```python
from build123d import *

# Parameters (mm, degrees)
SKETCH1_R           = 5
BOSS_EXTRUDE1_DEPTH = 10
SKETCH3_R           = 15
CUT_EXTRUDE2_DEPTH  = 2.5
SKETCH4_R           = 5
CUT_EXTRUDE3_DEPTH  = 74.484692283


with BuildPart() as part:
    # Sketch1 → Boss-Extrude1 (new, symmetric)
    with BuildSketch(Plane.XY):
        with BuildLine():
            Line((0, 10), (60, 10))
            ThreePointArc((60, 10), (70, 0), (60, -10))
            Line((60, -10), (0, -10))
            ThreePointArc((0, -10), (-10, 0), (0, 10))
        make_face()
        Circle(SKETCH1_R, mode=Mode.SUBTRACT)
        with Locations((60, 0)):
            Circle(SKETCH1_R, mode=Mode.SUBTRACT)
    extrude(amount=BOSS_EXTRUDE1_DEPTH, both=True)

    # Sketch3 → Cut-Extrude2 (cut, symmetric)
    with BuildSketch(Plane.XY):
        Circle(SKETCH3_R)
        with Locations((60, 0)):
            Circle(SKETCH3_R)
    extrude(amount=CUT_EXTRUDE2_DEPTH, both=True, mode=Mode.SUBTRACT)

    # Sketch4 → Cut-Extrude3 (cut, through all)
    with BuildSketch(Plane(origin=(0, 10, 0), x_dir=(1, 0, 0), z_dir=(0, 1, 0))):
        with Locations(Location((30, 0, 0), (0, 0, 270))):
            Circle(SKETCH4_R)
    extrude(amount=-CUT_EXTRUDE3_DEPTH, mode=Mode.SUBTRACT)


solid = part.part
```
Geometry check sheet. Reference: the model listing, model coordinates, mm. A direction names the side the tool comes from. Round coordinates to 2 decimals unless told otherwise and drop trailing zeros. Loops run counter-clockwise (first coordinate to the right, second up) from the corner with the lowest first, then second, coordinate; pieces in that order, holes last. Notation, with made-up numbers: (78, 41) - (84, 41) arc R27 cw to (84, 65) - close; hole circle Ø9 at (65.5, 72.5). An arc over 180 degrees is marked (long way). Write item = value, one per line. Start each with the question number.
1. Section check C-C on z = 0. Enter the section's corners in (x, y).
2. Section check B-B on x = 53.5. Enter the section's corners in (y, z).
3. Section check A-A on y = 0. Give the number of separate pieces and of enclosed holes in the cut face, then the cut area to 3 significant figures.
4. Section check D-D on z = -7.5. Enter the section's corners in (x, y), then the cut area to 3 significant figures.
5. Depth check by flat-ended pin: pin 1 (8 mm diameter, centred on y = 6, z = -4, fed in from +X); pin 2 (6 mm diameter, centred on x = 0, y = 0, fed in from +Z); pin 3 (8 mm diameter, centred on y = -4.5, z = -1.5, fed in from +X); pin 4 (8 mm diameter, centred on y = -7.5, z = -2, fed in from +X). Enter the tip coordinate at first touch or a pass-through.
6. Mould release check, pull along X, two halves, no side actions. Record for faces 3 (the face through (55, 0, 6)), 4 (the face through (15, 0, 0)), 5 (the face through (54.5, 0.1, -2.5)): released by +X, released by -X, zero draft, split by the parting line, or undercut.
7. Set-up check for faces 1 (the face through (-1.08, -4.88, -6.3)), 2 (the face through (45, 0, 0)): record each of +Z, -Z, +X, -X, +Y, -Y from which the full face is reachable in a straight line by a thin tool's end or side.
8. Thickness scan on line 1 (Z direction, x = 6.5, y = -4.75); line 2 (X direction, y = 0, z = -7); line 3 (Y direction, x = 0, z = -4.75). Record the ranges inside material, lowest first.
Working result:
q1.outline = (11.18, -10) - (25, -10) - (25, 10) - (11.18, 10) arc R15 cw to start; (35, -10) - (48.82, -10) arc R15 cw to (48.82, 10) - (35, 10) - close
q2.outline = (-10, -10) - (10, -10) - (10, -2.5) - (-10, -2.5) - close; (-10, 2.5) - (10, 2.5) - (10, 10) - (-10, 10) - close
q3.separate_pieces = 5
q3.enclosed_holes = 1
q3.area = 971 mm^2
q4.outline = (0, -10) - (60, -10) arc R10 ccw to (60, 10) - (0, 10) arc R10 ccw to start; hole circle Ø10 at (0, 0); hole circle Ø10 at (60, 0)
q4.area = 1,360 mm^2
q5.pin_1 = 69.8
q5.pin_2 = through
q5.pin_3 = 69.98
q5.pin_4 = 69.36
q6.face_3 = undercut
q6.face_4 = released by -X
q6.face_5 = zero draft
q7.face_1 = +Z, -Z
q7.face_2 = +X
q8.line_1 = -10 to -2.5, 2.5 to 10
q8.line_2 = -10 to -5, 5 to 55, 65 to 70
q8.line_3 = -10 to -5, 5 to 10
